```python
from build123d import *

# Parameters (mm, degrees)
F1_DEPTH      = 25
F2_W          = 29.447394362
F2_H          = 9.0000005439
F2_H_2        = 45.9999994561
F3_DEPTH      = 20
F4_W          = 4
F4_H          = 20
F5_DEPTH      = 50
F6_W          = 13.4000085294
F6_H          = 20
F6_W_2        = 12.5999914706
F7_DEPTH      = 47
F7_DEPTH_BACK = 10
F8_W          = 10
F8_H          = 10
F9_DEPTH      = 30
F10_R         = 5


with BuildPart() as f1:
    # F0 (on Front) → F1 (new body)
    with BuildSketch(Plane.XZ):
        Polygon((-89.7622789443, -41.3427457391), (40.2377210557, -41.3427457391), (40.2377210557, -41.1998914442), (40.2377210557, -21.8427457391), (-59.7622789443, -21.8427457391), (-59.7622789443, 58.1572542609), (-89.7622789443, 58.1572542609), align=None)
    extrude(amount=F1_DEPTH)

    # F2 (on face) → F3 (join)
    with BuildSketch(Plane.XY.offset(58.1572542609)):
        with Locations((-75.0385817632, -4.5000002719)):
            Rectangle(F2_W, F2_H)
        with Locations((-75.0385817632, 22.9999997281)):
            Rectangle(F2_W, F2_H_2)
    extrude(amount=-F3_DEPTH)

    # F4 (on face) → F5 (cut)
    with BuildSketch(Plane(origin=(0, 45.9999994561, 0), x_dir=(-1, 0, 0), z_dir=(0, 1, 0))):
        with Locations((75.038585484, 48.1572542609)):
            Rectangle(F4_W, F4_H)
    extrude(amount=-F5_DEPTH, mode=Mode.SUBTRACT)

    # F6 (on face) → F7 (join, two sides)
    with BuildSketch(Plane(origin=(0, 0, 0), x_dir=(-1, 0, 0), z_dir=(0, 1, 0))) as f7_sk:
        with Locations((66.462283209, 12.1572542609)):
            Rectangle(F6_W, F6_H)
        with Locations((83.462283209, 12.1572542609)):
            Rectangle(F6_W_2, F6_H)
    extrude(amount=F7_DEPTH)
    extrude(f7_sk.sketch, amount=-F7_DEPTH_BACK)

    # F8 (on face) → F9 (cut)
    with BuildSketch(Plane.YZ.offset(40.2377210557)):
        with Locations((-13, -31.3427457391)):
            Rectangle(F8_W, F8_H)
    extrude(amount=-F9_DEPTH, mode=Mode.SUBTRACT)

    # F10
    f10_edges = [f1.edges().sort_by_distance(p)[0] for p in [
        (-60.314885, 23, 58.157254),
        (-73.038585, 20.999999, 58.157254),
        (-60.314885, 23, 38.157254),
        (-73.038585, 23, 38.157254),
        (-77.038585, 23, 38.157254),
        (-89.762279, 23, 38.157254),
        (-89.762279, 10.5, 58.157254),
        (-77.038585, 20.999999, 58.157254),
        (-89.762279, 23.5, 2.157254),
        (-89.762279, 23.5, 22.157254),
        (-77.162287, 23.5, 22.157254),
        (-77.162287, 23.5, 2.157254),
        (-73.162287, 23.5, 2.157254),
        (-59.762279, 23.5, 2.157254),
        (-59.762279, 23.5, 22.157254),
        (-73.162287, 23.5, 22.157254),
        (-9.762279, 0, -21.842746),
        (-24.762279, 0, -41.342746),
        (-89.762279, 0, -19.592746),
        (-59.762279, 0, -9.842746),
        (-89.762279, -25, 8.407254),
        (-24.762279, -25, -41.342746),
        (-9.762279, -25, -21.842746),
        (-59.762279, -25, 18.157254),
    ]]
    fillet(f10_edges, radius=F10_R)


solid = f1.part
```
Verification items for the finished model (mm, model axes). A direction names the side the tool comes from. Give positions to 0.01 mm unless a question says otherwise; leave off trailing zeros. Order: outer loops, then holes, each group sorted by start corner. A loop starts at its lowest first (then second) coordinate and runs counter-clockwise, first axis right, second up. Notation, with made-up numbers: M -37,87.25 L -32,87.25 A15 ccw -32,102.25 Z; hole C 9.5,57 d2. An arc over 180 degrees is marked long. Return JSON: item names as keys, results as strings. Group by question number.
1) Go/stop test with flat-tipped pins: pin 1 Ø0.8 at (x, y) = (-83.5, 25) entering from -Z; pin 2 Ø8 at (y, z) = (24, -2.5) entering from -X; pin 3 Ø4 at (x, z) = (-66.5, 44.5) entering from +Y; pin 4 Ø8 at (y, z) = (32, 48) entering from +X. Record where each tip stops, or that it passes through.
2) Section check C-C on z = -19. Record the cut outline in (x, y), and give its area (3 significant figures).
3) Section check D-D on y = -12.5. Record the cut outline in (x, z), and give its area (3 significant figures).
4) Mould release check, pull along X, two halves, no side actions. Record for faces 5 (the face through (-78.54, 20.65, 56.73)), 6 (the face through (-13, -23.5, -23.27)), 7 (the face through (-59.762, -1, 18)): pulls with the +X half, pulls with the -X half, needs draft (parallel to the pull), parting line crosses it, or undercut.
5) Section check B-B on y = 30. Give the number of separate pieces and of enclosed holes in the cut face, and give its area (3 significant figures).
6) Section check A-A on x = 23. Record the cut outline in (y, z), and give its area (3 significant figures).
7) Access from +Z, -Z, +X, -X, +Y, -Y to the whole of each face (thin tool, end or side, straight path). Record for faces 1 (the face through (-61.19, -1.5, -9.6)), 2 (the face through (-73.162, 23, 12)), 3 (the face through (-67, 46, 48)), 4 (the face through (-78.67, 23.83, 3.58)).
8) Scan lines: line 1 (X direction, y = -2, z = 44.5); line 2 (Z direction, x = 16.5, y = -13); line 3 (X direction, y = 27, z = 10). Record each from-to range of solid material in increasing order.
Answer block:
{
 "1": {"pin 1": "stops at z = 2.16", "pin 2": "passes through", "pin 3": "stops at y = 46", "pin 4": "stops at x = -60.31"},
 "2": {"outline": "M -89.76,-20 A5 ccw -84.76,-25 L -64.76,-25 A5 ccw -59.76,-20 L -59.76,-5 A5 ccw -64.76,0 L -84.76,0 A5 ccw -89.76,-5 Z", "area": "729 mm^2"},
 "3": {"outline": "M -89.76,-41.34 L 40.24,-41.34 L 40.24,-36.34 L 10.24,-36.34 L 10.24,-26.34 L 40.24,-26.34 L 40.24,-21.84 L -59.76,-21.84 L -59.76,58.16 L -84.76,58.16 A5 ccw -89.76,53.16 Z", "area": "4,630 mm^2"},
 "4": {"face 5": "undercut", "face 6": "needs draft", "face 7": "pulls with the +X half"},
 "5": {"separate pieces": "4", "enclosed holes": "0", "area": "943 mm^2"},
 "6": {"outline": "M -25,-36.34 A5 ccw -20,-41.34 L -5,-41.34 A5 ccw 0,-36.34 L 0,-26.84 A5 ccw -5,-21.84 L -20,-21.84 A5 ccw -25,-26.84 Z; hole M -18,-36.34 L -8,-36.34 L -8,-26.34 L -18,-26.34 Z", "area": "366 mm^2"},
 "7": {"face 1": "+X, +Y", "face 2": "+Z, -Z, +Y", "face 3": "+Z, +X, -X, +Y", "face 4": "-Z, +Y"},
 "8": {"line 1": "x = -89.76 to -77.04, -73.04 to -59.76", "line 2": "z = -41.34 to -36.34, -26.34 to -21.84", "line 3": "x = -89.76 to -77.16, -73.16 to -59.76"}
}
